Answer from the drawing. Dimensions are ordinates in mm from the lowest x, y and z of the part. Coordinates: 2 decimals unless noted, no trailing zeros. Loops run counter-clockwise (first coordinate to the right, second up) from the corner with the lowest first, then second, coordinate; pieces in that order, holes last. Notation, with made-up numbers: (66.25, -34.75) -> (73.25, -34.75) arc R5 cw to (73.25, -28.75) -> close; hole circle Ø5 at (17.25, 13). An arc over 180 degrees is marked (long way). Use a Markdown table: item, result.
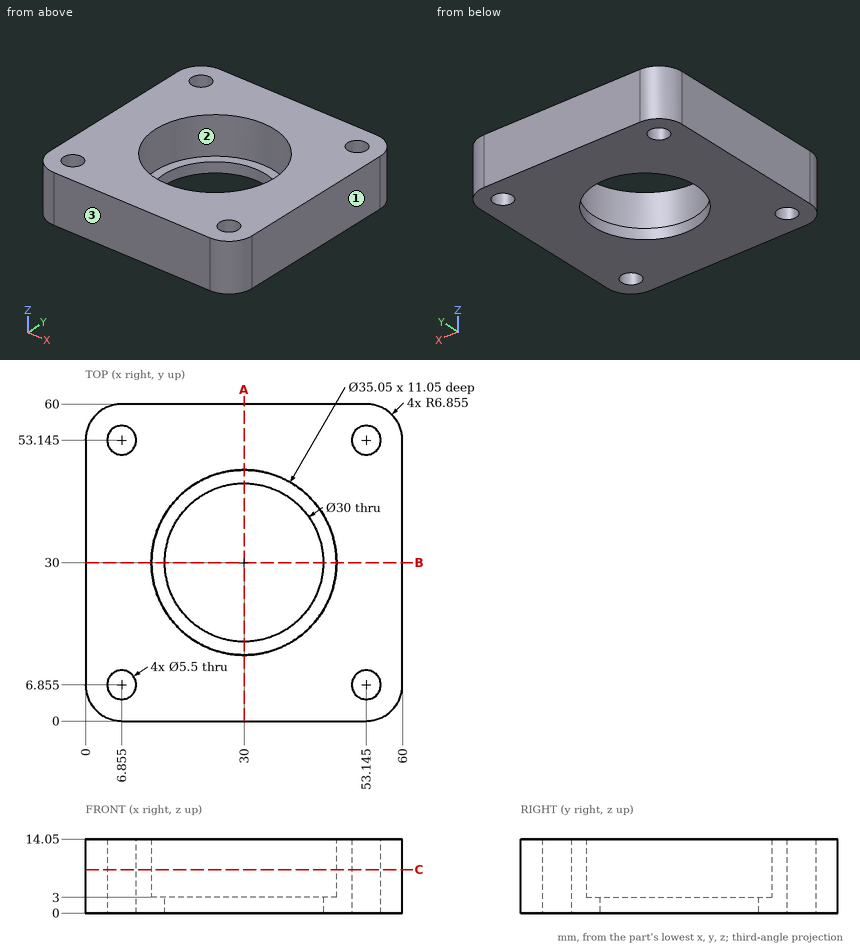
Q1. Section A-A on x = 30 is taken. Determine the outline of the cut face in (y, z) (3 decimals).
Solved:
| item | result |
|---|---|
| outline | (0, 0) -> (15, 0) -> (15, 3) -> (12.475, 3) -> (12.475, 14.05) -> (0, 14.05) -> close; (45, 0) -> (60, 0) -> (60, 14.05) -> (47.525, 14.05) -> (47.525, 3) -> (45, 3) -> close |
Q2. Determine the mould class of the marked faces 1, 2 and 3 for opening direction X: pulls with the +X half, pulls with the -X half, needs draft (parallel to the pull), parting line crosses it, or undercut.
Solved:
| item | result |
|---|---|
| face 1 | pulls with the +X half |
| face 2 | undercut |
| face 3 | needs draft |
Q3. Section C-C on z = 8.25 is taken. Determine the outline of the cut face in (x, y) (3 decimals).
Solved:
| item | result |
|---|---|
| outline | (0, 6.855) arc R6.855 ccw to (6.855, 0) -> (53.145, 0) arc R6.855 ccw to (60, 6.855) -> (60, 53.145) arc R6.855 ccw to (53.145, 60) -> (6.855, 60) arc R6.855 ccw to (0, 53.145) -> close; hole circle Ø5.5 at (6.855, 6.855); hole circle Ø5.5 at (6.855, 53.145); hole circle Ø35.05 at (30, 30); hole circle Ø5.5 at (53.145, 6.855); hole circle Ø5.5 at (53.145, 53.145) |
Q4. Consider line 1 (Y direction, x = 54.5, z = 12); line 2 (Y direction, x = 5, z = 11.5); line 3 (X direction, y = 8.5, z = 1.5). Determine where each line is inside the solid, lowest interval first. Write a range as [from, to].
Solved:
| item | result |
|---|---|
| line 1 | [0.14, 4.46], [9.25, 50.75], [55.54, 59.86] |
| line 2 | [0.26, 4.82], [8.89, 51.11], [55.18, 59.74] |
| line 3 | [0, 4.65], [9.06, 50.94], [55.35, 60] |
